Source: three-view drawing plus pictorial views. Frame: mm from the lowest corner of the part. A direction names the side the tool comes from. Round coordinates to 2 decimals unless told otherwise and drop trailing zeros. Loops run counter-clockwise (first coordinate to the right, second up) from the corner with the lowest first, then second, coordinate; pieces in that order, holes last. Notation, with made-up numbers: (27, 9) -> (32, 9) arc R14 ccw to (32, 13) -> close; hole circle Ø2 at (-23.5, -21.75). An arc over 180 degrees is marked (long way). Put each result on its own line as item: value. Start each with the question number.
1. Set-up query: the marked faces 4 and 5. Return all of +Z, -Z, +X, -X, +Y, -Y with unobstructed straight access to the full face (end or side cutting, diameter ignored); none if empty.
2. Cut plane B-B (x = 1.75). Return the cut outline in (y, z), then the cut area to 3 significant figures.
3. Cut plane A-A (z = 1). Return the cut outline in (x, y).
4. Cut plane D-D (z = 6.75). Return the cut outline in (x, y).
5. Contact query for flat-ended pins moving along their axis: pin 1 (0.8 mm diameter, centred on x = 2.5, y = 1.5, fed in from -Z); pin 2 (2 mm diameter, centred on x = 2, z = 8.5, fed in from -Y). Output: stop coordinate, or through.
6. Draft query along Y for the marked faces 1, 2 and 3. Return one class per face: pulls with the +Y half, pulls with the -Y half, needs draft (parallel to the pull), parting line crosses it, or undercut.
7. Material intervals for L1, parallel to Z at x = 1.6, y = 1.8; L2, parallel to Z at x = 2.4, y = 0.55; L3, parallel to Y at x = 2, z = 0.75, sorted ascending.
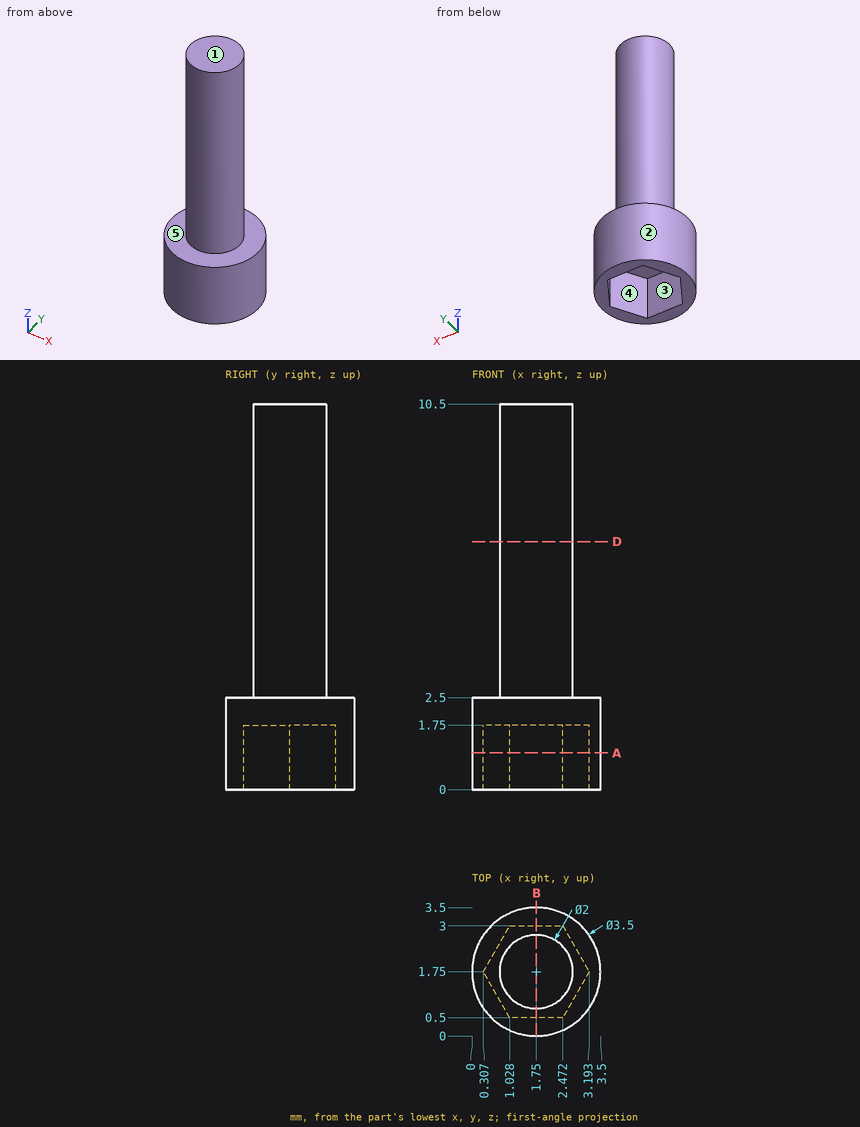
Solution:
1. face 4: -Z
1. face 5: +Z
2. outline: (0, 0) -> (0.5, 0) -> (0.5, 1.75) -> (3, 1.75) -> (3, 0) -> (3.5, 0) -> (3.5, 2.5) -> (2.75, 2.5) -> (2.75, 10.5) -> (0.75, 10.5) -> (0.75, 2.5) -> (0, 2.5) -> close
2. area: 20.4 mm^2
3. outline: circle Ø3.5 at (1.75, 1.75); hole (0.31, 1.75) -> (1.03, 0.5) -> (2.47, 0.5) -> (3.19, 1.75) -> (2.47, 3) -> (1.03, 3) -> close
4. outline: circle Ø2 at (1.75, 1.75)
5. pin 1: stops at z = 1.75
5. pin 2: stops at y = 0.75
6. face 1: needs draft
6. face 2: parting line crosses it
6. face 3: undercut
7. L1: z = 1.75 to 10.5
7. L2: z = 1.75 to 2.5
7. L3: y = 0.02 to 0.5, 3 to 3.48
